Can you work these out from the drawing? Everything is in mm from the part's minimum corner. Give positions to 0.01 mm unless a question says otherwise; leave off trailing zeros. Loops run counter-clockwise (first coordinate to the right, second up) from the corner with the lowest first, then second, coordinate; pieces in that order, holes last. Notation, with made-up numbers: (-19, -7) - (-11, -7) arc R30 cw to (-11, 22) - close; hole circle Ø7 at (16.5, 84). An arc over 180 degrees is marked (long way). Answer in a Markdown table with one row per item.
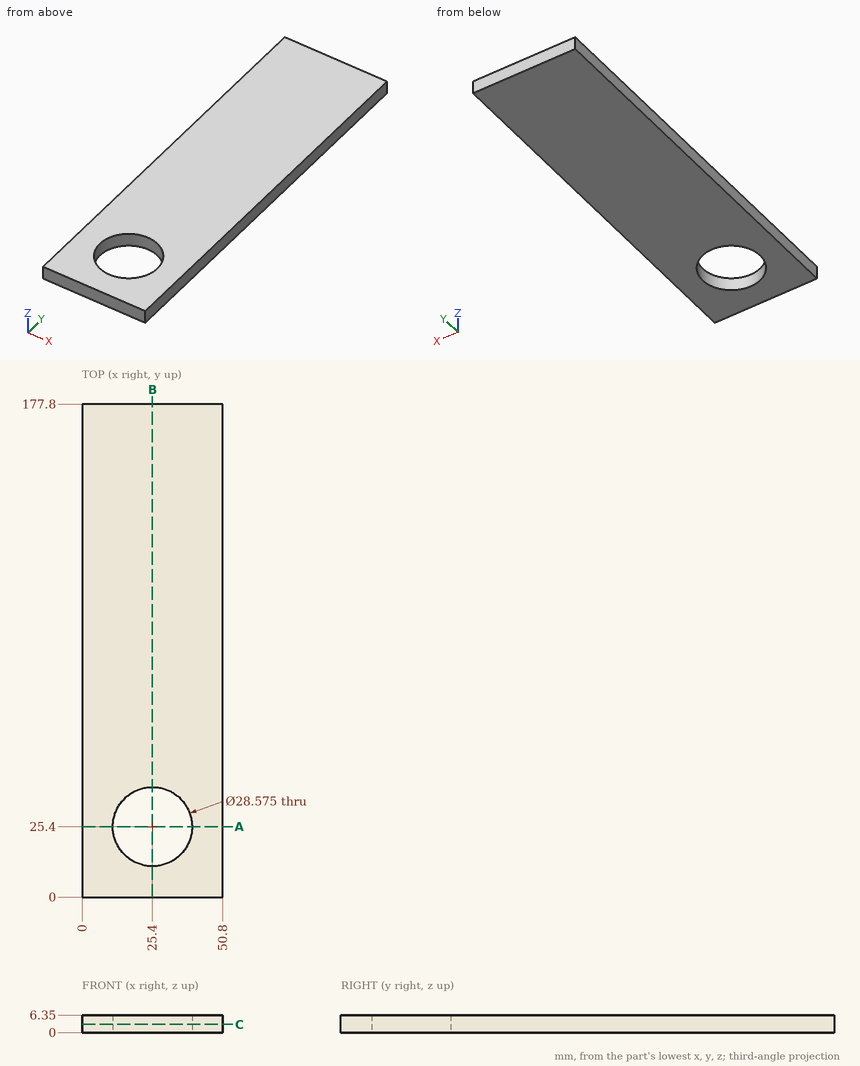
Q1. If I drill on line 1 (Y direction, x = 25.4, z = 4); line 2 (X direction, y = 25.4, z = 4.5); line 3 (X direction, y = 17, z = 2.25), over which ranges is the centre line in solid material (lowest first)? Write a range as [from, to].
Checked values:
| item | result |
|---|---|
| line 1 | y = [0, 11.11], [39.69, 177.8] |
| line 2 | x = [0, 11.11], [39.69, 50.8] |
| line 3 | x = [0, 13.84], [36.96, 50.8] |
Q2. Imagine slicing it at A-A, the plane y = 25.4. Write out the boundary of the cut face in (x, z), and give its area (3 significant figures).
Checked values:
| item | result |
|---|---|
| outline | (0, 0) - (11.11, 0) - (11.11, 6.35) - (0, 6.35) - close; (39.69, 0) - (50.8, 0) - (50.8, 6.35) - (39.69, 6.35) - close |
| area | 141 mm² |
Q3. Imagine slicing it at C-C, the plane z = 3. Write out the boundary of the cut face in (x, y) (1 decimal), and give its area (3 significant figures).
Checked values:
| item | result |
|---|---|
| outline | (0, 0) - (50.8, 0) - (50.8, 177.8) - (0, 177.8) - close; hole circle Ø28.6 at (25.4, 25.4) |
| area | 8,390 mm² |
Q4. Imagine slicing it at B-B, the plane x = 25.4. Write out the boundary of the cut face in (y, z), and give its area (3 significant figures).
Checked values:
| item | result |
|---|---|
| outline | (0, 0) - (11.11, 0) - (11.11, 6.35) - (0, 6.35) - close; (39.69, 0) - (177.8, 0) - (177.8, 6.35) - (39.69, 6.35) - close |
| area | 948 mm² |
